Print and shaded views of the part. All mm, measured from the part's lowest x, y and z. A direction names the side the tool comes from. Give positions to 0.01 mm unless a question says otherwise; leave off trailing zeros. Loops run counter-clockwise (first coordinate to the right, second up) from the corner with the lowest first, then second, coordinate; pieces in that order, holes last. Notation, with made-up numbers: M 56.5,87 L 73.5,87 A28 ccw 73.5,123 Z; hole C 17.5,13.25 d9. An arc over 180 degrees is marked long. Answer in a Markdown table with one row per item.
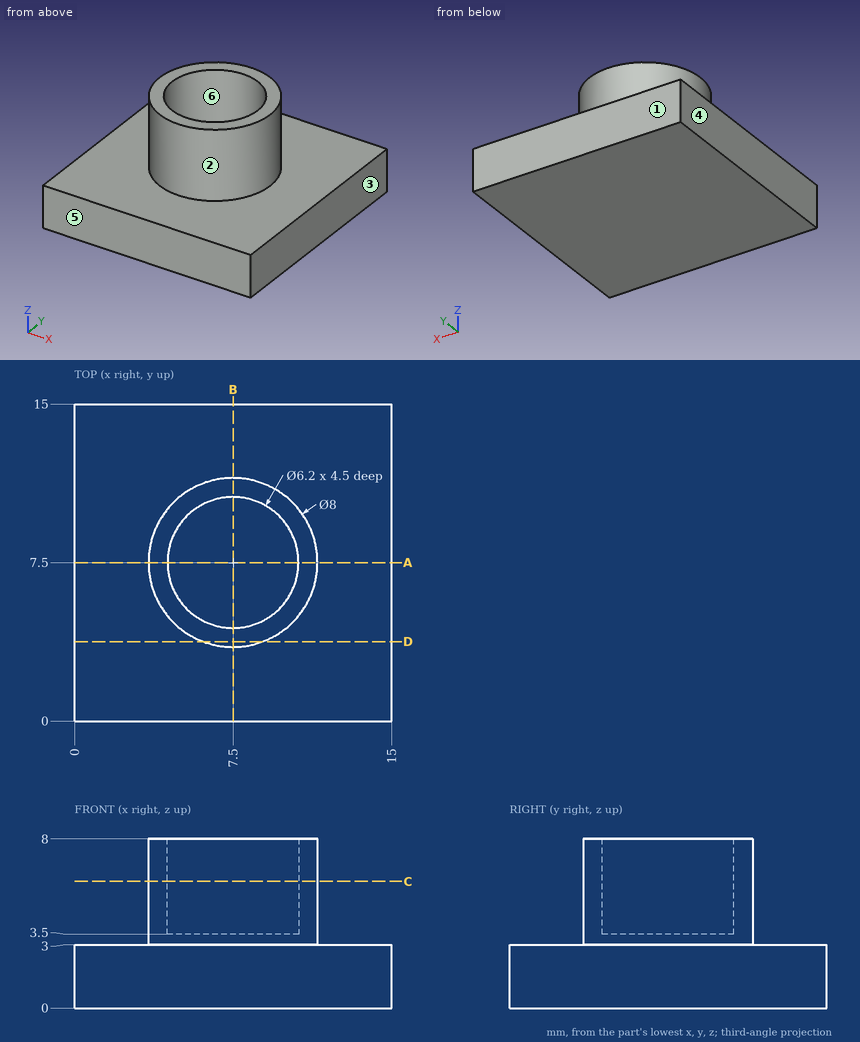
(1) Saw through at C-C, the plane z = 6. Give the cut face in (x, y).
Established:
| item | result |
|---|---|
| outline | C 7.5,7.5 d8; hole C 7.5,7.5 d6.2 |
(2) Which spindle directions (+Z, -Z, +X, -X, +Y, -Y) get a long thin tool onto all of the face, cutting with end or side? Do the marked faces 1 and 2. Say none if no direction does.
Established:
| item | result |
|---|---|
| face 1 | +Z, -Z, +X, -X, +Y |
| face 2 | +Z |
(3) Saw through at A-A, the plane y = 7.5. Give the cut face in (x, z), and give its area (3 significant figures).
Established:
| item | result |
|---|---|
| outline | M 0,0 L 15,0 L 15,3 L 11.5,3 L 11.5,8 L 10.6,8 L 10.6,3.5 L 4.4,3.5 L 4.4,8 L 3.5,8 L 3.5,3 L 0,3 Z |
| area | 57.1 mm2 |
(4) Mould opens along X. For the marked faces 3, 4, 5 and 6 say: pulls with the +X half, pulls with the -X half, needs draft (parallel to the pull), parting line crosses it, or undercut.
Established:
| item | result |
|---|---|
| face 3 | pulls with the +X half |
| face 4 | pulls with the -X half |
| face 5 | needs draft |
| face 6 | undercut |
(5) Flat gauge pins, fed straight in: P1, Ø3, axis at y = 12.5, z = 6.5, coming from the +X side; P2, Ø1.5, axis at y = 8, z = 5.5, coming from the -X side; P3, Ø4, axis at x = 2.5, y = 8, coming from the -Z side; P4, Ø5, axis at x = 7.5, y = 7.5, coming from the +Z side. Where does each tip first touch, or does it go through?
Established:
| item | result |
|---|---|
| P1 | stops at x = 9.44 |
| P2 | stops at x = 3.5 |
| P3 | stops at z = 0 |
| P4 | stops at z = 3.5 |
(6) Wall check: L1, parallel to Y at x = 7.5, z = 5.65; L2, parallel to Z at x = 5.75, y = 5.5; L3, parallel to Z at x = 13.75, y = 11.75. Give the ranges that are in metal, low to high.
Established:
| item | result |
|---|---|
| L1 | y = 3.5 to 4.4, 10.6 to 11.5 |
| L2 | z = 0 to 3.5 |
| L3 | z = 0 to 3 |
(7) Saw through at D-D, the plane y = 3.75. Give the cut face in (x, z), and give its area (3 significant figures).
Established:
| item | result |
|---|---|
| outline | M 0,0 L 15,0 L 15,3 L 8.89,3 L 8.89,8 L 6.11,8 L 6.11,3 L 0,3 Z |
| area | 58.9 mm2 |
